For this review, take the finished solid that the model builds, in its own axes (mm). A direction names the side the tool comes from. Give positions to 0.01 mm unless a question says otherwise; leave off trailing zeros. Order: outer loops, then holes, each group sorted by start corner. A loop starts at its lowest first (then second) coordinate and runs counter-clockwise, first axis right, second up. Notation, with made-up numbers: (24.5, 38.25) -> (64.5, 38.25) arc R20 ccw to (64.5, 72.25) -> close; hole circle Ø8 at (49, 23). An arc over 180 degrees is marked (long way). Use CSV: the item, a comma, the result in double quotes. Start each with the question number.
```python
from build123d import *

# Parameters (mm, degrees)
SKETCH_1_R          = 15
SKETCH_1_R_2        = 13
EXTRUDE_1_DEPTH     = 90
EXTRUDE_START       = 10
SKETCH_2_R          = 15
EXTRUDE_2_DEPTH     = 10
CUT_EXTRUDE_1_DEPTH = 4
SKETCH_4_R          = 3.25
CUT_EXTRUDE_2_DEPTH = 97.363893653


with BuildPart() as part:
    # Эскиз1 → Бобышка-Вытянуть1 (new body)
    with BuildSketch(Plane(origin=(0, 0, 0), x_dir=(1, 0, 0), z_dir=(0, 1, 0))):
        with Locations(Location((0, 0, 0), (0, 0, 90))):
            Circle(SKETCH_1_R)
        with Locations(Location((0, 0, 0), (0, 0, 90))):
            Circle(SKETCH_1_R_2, mode=Mode.SUBTRACT)
    extrude(amount=EXTRUDE_1_DEPTH)

    # Эскиз2 → Бобышка-Вытянуть2 (add)
    with BuildSketch(Plane.XZ.offset(EXTRUDE_START)):
        with Locations(Location((0, 0, 0), (0, 0, 270))):
            Circle(SKETCH_2_R)
    extrude(amount=-EXTRUDE_2_DEPTH)

    # Эскиз3 → Вырез-Вытянуть1 (cut)
    with BuildSketch(Plane(origin=(0, 0, 0), x_dir=(1, 0, 0), z_dir=(0, 1, 0))):
        Polygon((2.886751346, 5), (-2.886751346, 5), (-5.773502692, 0), (-2.886751346, -5), (2.886751346, -5), (5.773502692, 0), align=None)
    extrude(amount=-CUT_EXTRUDE_1_DEPTH, mode=Mode.SUBTRACT)

    # Эскиз4 → Вырез-Вытянуть2 (cut, through all)
    with BuildSketch(Plane(origin=(0, -4, 0), x_dir=(1, 0, 0), z_dir=(0, 1, 0))):
        with Locations(Location((0, 0, 0), (0, 0, 270))):
            Circle(SKETCH_4_R)
    extrude(amount=-CUT_EXTRUDE_2_DEPTH, mode=Mode.SUBTRACT)


solid = part.part
```
1. Consider section D-D (z = 9). State the section outline as (x, y) points.
2. To check wall thickness, follow L1, parallel to X at y = -5.55, z = 0; L2, parallel to X at y = 55, z = 0; L3, parallel to Z at x = 4.75, y = 38. State the ranges of each line that lie inside material, in increasing order. Write a range as [from, to].
3. Consider section C-C (z = -12). State the section outline as (x, y) points.
4. Consider section A-A (x = 0). State the section outline as (y, z) points.
5. For faces 4 (the face through (-1.978, -6.958, -2.579)), 5 (the face through (0, -2, -5)), list the 3-axis set-ups (+Z, -Z, +X, -X, +Y, -Y) from which the entire face can be reached by the end or side of a thin tool; tool diameter is ignored.
6. Consider section B-B (y = 27). State the section outline as (x, z) points, plus the area to 3 significant figures.
7. Draft analysis for pull direction X (two halves, no side actions). For faces 1 (the face through (-4.35, -1.972, 2.465)), 2 (the face through (-13.4, 90, 0.1)), 3 (the face through (0.66, 39.3, 14.985)), state which applies: +X half, -X half, draft (parallel to the pull), parting line (faces both ways), or undercut.
8. Clearance check with flat-ended pins moving along their axes: P1, Ø1, axis at x = -10.5, z = 2.5, coming from the +Y side; P2, Ø1, axis at y = 21.5, z = 8.5, coming from the +X side; P3, Ø1.5, axis at x = 11.5, y = 40.5, coming from the +Z side. State where each tip first meets the part, or that it passes through.
Answer list:
1,outline,"(-12, -10) -> (12, -10) -> (12, 90) -> (9.38, 90) -> (9.38, 0) -> (-9.38, 0) -> (-9.38, 90) -> (-12, 90) -> close"
2,L1,"[-15, -3.25], [3.25, 15]"
2,L2,"[-15, -13], [13, 15]"
2,L3,"[-14.23, -12.1], [12.1, 14.23]"
3,outline,"(-9, -10) -> (9, -10) -> (9, 90) -> (5, 90) -> (5, 0) -> (-5, 0) -> (-5, 90) -> (-9, 90) -> close"
4,outline,"(-10, -15) -> (90, -15) -> (90, -13) -> (0, -13) -> (0, -5) -> (-4, -5) -> (-4, -3.25) -> (-10, -3.25) -> close; (-10, 3.25) -> (-4, 3.25) -> (-4, 5) -> (0, 5) -> (0, 13) -> (90, 13) -> (90, 15) -> (-10, 15) -> close"
5,face 4,"+Y, -Y"
5,face 5,"+Y"
6,outline,"circle Ø30 at (0, 0); hole circle Ø26 at (0, 0)"
6,area,"176 mm2"
7,face 1,"undercut"
7,face 2,"draft"
7,face 3,"parting line"
8,P1,"y = 0"
8,P2,"x = 12.69"
8,P3,"z = 10.46"
